Study the drawing (mm; zero at the part's minimum x, y, z) and answer. Coordinates: 2 decimals unless noted, no trailing zeros. Loops run counter-clockwise (first coordinate to the right, second up) from the corner with the lowest first, then second, coordinate; pieces in that order, holes last. Notation, with made-up numbers: (-38.5, -15) -> (-1.5, -15) arc R27 cw to (-1.5, 11) -> close; hole circle Ø4 at (-33.5, 78). An arc over 180 degrees is marked (long way). Answer in a Markdown table with one row per item.
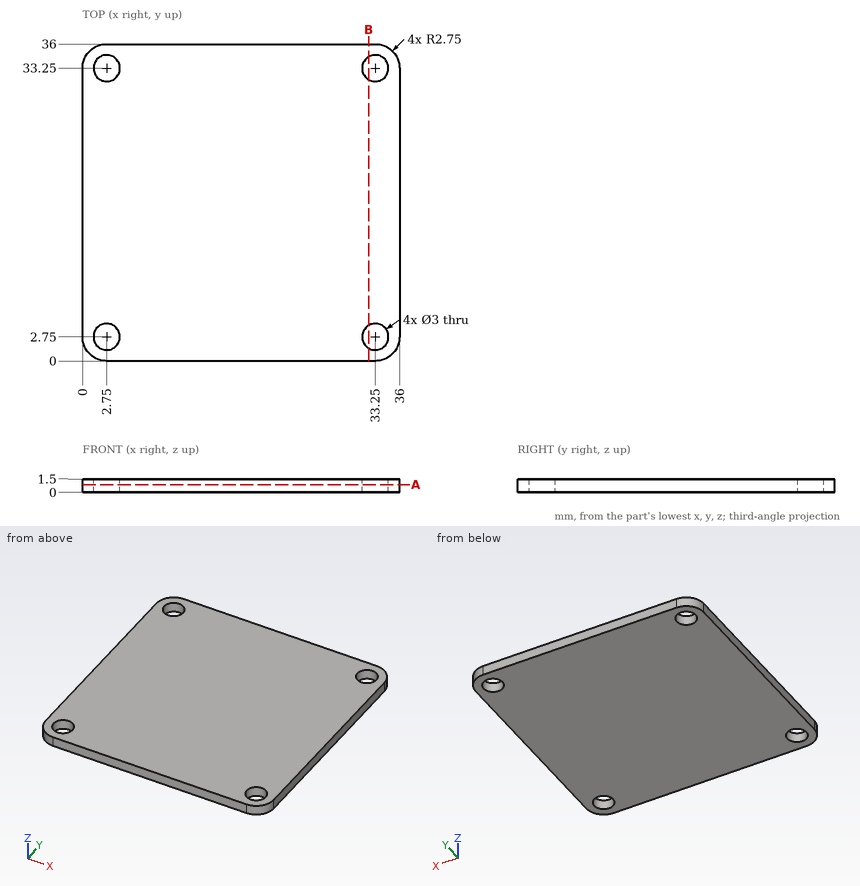
1. A cutting plane is placed at B-B on x = 32.5. Give the vertices of the cut face in (y, z), and give its area (3 significant figures).
A:
| item | result |
|---|---|
| outline | (0, 0) -> (1.45, 0) -> (1.45, 1.5) -> (0, 1.5) -> close; (4.05, 0) -> (31.95, 0) -> (31.95, 1.5) -> (4.05, 1.5) -> close; (34.55, 0) -> (36, 0) -> (36, 1.5) -> (34.55, 1.5) -> close |
| area | 46.2 mm2 |
2. A cutting plane is placed at A-A on z = 0.85. Give the vertices of the cut face in (x, y), and give its area (3 significant figures).
A:
| item | result |
|---|---|
| outline | (0, 2.75) arc R2.75 ccw to (2.75, 0) -> (33.25, 0) arc R2.75 ccw to (36, 2.75) -> (36, 33.25) arc R2.75 ccw to (33.25, 36) -> (2.75, 36) arc R2.75 ccw to (0, 33.25) -> close; hole circle Ø3 at (2.75, 2.75); hole circle Ø3 at (2.75, 33.25); hole circle Ø3 at (33.25, 2.75); hole circle Ø3 at (33.25, 33.25) |
| area | 1,260 mm2 |
3. Find the intervals of material crossed by probe 1 along Y at (x, z) = (2.75, 1.05); probe 2 along X at (y, z) = (32.5, 0.65), in increasing order.
A:
| item | result |
|---|---|
| probe 1 | y = 0 to 1.25, 4.25 to 31.75, 34.75 to 36 |
| probe 2 | x = 0 to 1.45, 4.05 to 31.95, 34.55 to 36 |
